Part model, mm, in its own coordinate system. Give positions to 0.01 mm unless a question says otherwise; leave off trailing zeros. Order: outer loops, then holes, each group sorted by start corner. A loop starts at its lowest first (then second) coordinate and runs counter-clockwise, first axis right, second up.
1. Slice it at C-C on y = 1.4. List the corners of the cut face in (x, z) (1 decimal).
2. Drop a flat-ended pin along its axis: pin 1 Ø2 at (x, z) = (29.5, 19) entering from -Y. Give the stop position or say it passes through.
3. Slice it at A-A on x = -82.67. List the corners of the cut face in (y, z) (1 decimal).
4. Probe line 1 (X direction, y = 1, z = -7); line 2 (Z direction, x = -82.67, y = 1.25) (1 decimal); line 3 (X direction, y = 1.7, z = 15.5). List the from-to ranges inside material, lowest first.
5. Slice it at B-B on z = -3.5. List the corners of the cut face in (x, y), and give its area (3 significant figures).
from build123d import *

# Parameters (mm, degrees)
SCHIZZO1_W                   = 180.34
SCHIZZO1_H                   = 48.45
ESTRUSIONE_ESTRUSIONE1_DEPTH = 3
SCHIZZO2_R                   = 1.5
SCHIZZO2_W                   = 5
SCHIZZO2_H                   = 15
TAGLIO_ESTRUSIONE1_DEPTH     = 4


with BuildPart() as part:
    # Schizzo1 → Estrusione-Estrusione1 (new body)
    with BuildSketch(Plane(origin=(0, 0, 0), x_dir=(1, 0, 0), z_dir=(0, 1, 0))):
        Rectangle(SCHIZZO1_W, SCHIZZO1_H)
    extrude(amount=ESTRUSIONE_ESTRUSIONE1_DEPTH)

    # Schizzo2 → Taglio-Estrusione1 (cut, through all)
    with BuildSketch(Plane(origin=(0, 0, 0), x_dir=(1, 0, 0), z_dir=(0, 1, 0))):
        with Locations((-82.67, -15.8625)):
            Circle(SCHIZZO2_R)
        with Locations((82.67, -15.8625)):
            Circle(SCHIZZO2_R)
        with Locations((-82.67, 0)):
            Rectangle(SCHIZZO2_W, SCHIZZO2_H)
        with Locations((82.67, 0)):
            Rectangle(SCHIZZO2_W, SCHIZZO2_H)
    extrude(amount=TAGLIO_ESTRUSIONE1_DEPTH, mode=Mode.SUBTRACT)


solid = part.part
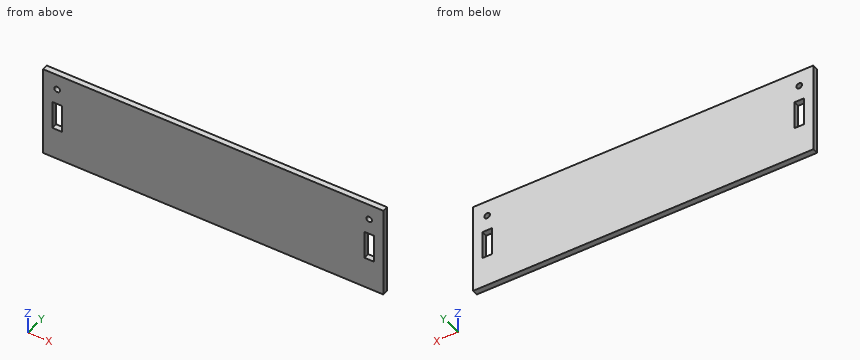
Data:
1. outline: (-90.2, -24.2) - (90.2, -24.2) - (90.2, 24.2) - (-90.2, 24.2) - close; hole (-85.2, -7.5) - (-80.2, -7.5) - (-80.2, 7.5) - (-85.2, 7.5) - close; hole circle Ø3 at (-82.7, 15.9); hole (80.2, -7.5) - (85.2, -7.5) - (85.2, 7.5) - (80.2, 7.5) - close; hole circle Ø3 at (82.7, 15.9)
2. pin 1: stops at y = 0
3. outline: (0, -24.2) - (3, -24.2) - (3, -7.5) - (0, -7.5) - close; (0, 7.5) - (3, 7.5) - (3, 14.4) - (0, 14.4) - close; (0, 17.4) - (3, 17.4) - (3, 24.2) - (0, 24.2) - close
4. line 1: x = -90.17 to -85.17, -80.17 to 80.17, 85.17 to 90.17
4. line 2: z = -24.2 to -7.5, 7.5 to 14.4, 17.4 to 24.2
4. line 3: x = -90.17 to -84.13, -81.21 to 81.21, 84.13 to 90.17
5. outline: (-90.17, 0) - (-85.17, 0) - (-85.17, 3) - (-90.17, 3) - close; (-80.17, 0) - (80.17, 0) - (80.17, 3) - (-80.17, 3) - close; (85.17, 0) - (90.17, 0) - (90.17, 3) - (85.17, 3) - close
5. area: 511 mm2
